Here's how the part is built. I have some questions about the finished solid (model axes, mm). A direction names the side the tool comes from. Coordinates: 2 decimals unless noted, no trailing zeros. Order: outer loops, then holes, each group sorted by start corner. A loop starts at its lowest first (then second) coordinate and runs counter-clockwise, first axis right, second up. Notation, with made-up numbers: (76.25, 47.25) - (106.25, 47.25) arc R20 ccw to (106.25, 83.25) - close; hole circle Ø8 at (-20, 68.5). An arc over 180 degrees is marked (long way). Answer in a Markdown table with one row per item. Add a question column.
Item 1: Will these pins go through, and if not, where does the flat tip stop? pin 1 Ø0.8 at (y, z) = (1, 32) entering from -X; pin 2 Ø1.5 at (x, z) = (-7.5, 0.5) entering from +Y; pin 3 Ø0.6 at (x, y) = (-6, -0.5) entering from +Z; pin 4 Ø1 at (y, z) = (-0.5, -5) entering from +X (3 decimals).
Item 2: I want a section at A-A (x = -10). Please give me the cut outline in (y, z), plus the area to 3 significant figures.
Item 3: On a 3-axis mill with a long thin cutter (end or side, diameter ignored), from which of +Z, -Z, +X, -X, +Y, -Y can I reach the whole of each face in a straight line? I mean faces 1 (the flat face through (-20, 1, 70.612)), 2 (the flat face through (-27.773, -0.626, 26.551)), 3 (the flat face through (-20, -1.27, 35)). Say none if no direction works.
Item 4: I want a section at D-D (y = -0.6). Count the separate pieces of the cut face and the enclosed holes in it, plus the area to 3 significant figures.
Item 5: If I drill on line 1 along X through (y, z) = (2.05, 52); line 2 along X through (y, z) = (-0.9, -7.62) (1 decimal); line 3 along Z through (x, y) = (-27.5, 0.55), over which ranges is the centre line in solid material (lowest first)? Write a range as from..to.
Item 6: Thinking about a two-plate mould opening in X: for faces 4 (the flat face through (-20, 1, -1.27)), 5 (the flat face through (-40.64, 1, 35)), 6 (the cylindrical face through (-20.03, -0.63, -6.07)), which applies, +X half, -X half, draft (parallel to the pull), parting line (faces both ways), or undercut?
Item 7: I want a section at B-B (z = 61). Please give me the cut outline in (x, y), plus the area to 3 significant figures.
Item 8: I want a section at C-C (x = -3.5). Please give me the cut outline in (y, z).
```python
from build123d import *

# Parameters (mm, degrees)
SKETCH1_W           = 41.91
SKETCH1_H           = 71.882
SKETCH1_W_2         = 39.37
SKETCH1_H_2         = 69.342
BOSS_EXTRUDE4_DEPTH = 2.54
SKETCH5_W           = 46.99
SKETCH5_H           = 76.962
BOSS_EXTRUDE5_DEPTH = 1.27
CHAMFER4_SIZE       = 2.54
CUT_EXTRUDE1_DEPTH  = 2.54
FILLET1_R           = 2.54
SKETCH7_R           = 1.5875
BOSS_EXTRUDE6_DEPTH = 1.27


with BuildPart() as part:
    # Sketch1 → Boss-Extrude4 (new body)
    with BuildSketch(Plane(origin=(0, 0, 0), x_dir=(1, 0, 0), z_dir=(0, 1, 0))):
        with Locations((-19.685, -34.671)):
            Rectangle(SKETCH1_W, SKETCH1_H)
        with Locations((-19.685, -34.671)):
            Rectangle(SKETCH1_W_2, SKETCH1_H_2, mode=Mode.SUBTRACT)
    extrude(amount=BOSS_EXTRUDE4_DEPTH)

    # Sketch5 → Boss-Extrude5 (add)
    with BuildSketch(Plane.XZ):
        with Locations((-19.685, 34.671)):
            Rectangle(SKETCH5_W, SKETCH5_H)
    extrude(amount=BOSS_EXTRUDE5_DEPTH)

    # Chamfer4
    chamfer4_edges = [part.edges().sort_by_distance(p)[0] for p in [
        (-43.18, -0.635, 73.152),
        (-43.18, -0.635, -3.81),
        (3.81, -0.635, -3.81),
        (3.81, -0.635, 73.152),
    ]]
    chamfer(chamfer4_edges, length=CHAMFER4_SIZE)

    # Sketch6 → Cut-Extrude1 (cut)
    with BuildSketch(Plane(origin=(0, 0, 0), x_dir=(1, 0, 0), z_dir=(0, 1, 0))):
        Polygon((-36.83, -2.54), (-2.54, -2.54), (-19.685, -29.888964801), align=None)
        Polygon((-36.83, -12.104070398), (-36.83, -57.237929602), (-22.68284632, -34.671), align=None)
        Polygon((-36.83, -66.802), (-2.54, -66.802), (-19.685, -39.453035199), align=None)
        Polygon((-2.54, -12.104070398), (-2.54, -57.237929602), (-16.68715368, -34.671), align=None)
    extrude(amount=-CUT_EXTRUDE1_DEPTH, mode=Mode.SUBTRACT)

    # Fillet1
    fillet1_edges = [part.edges().sort_by_distance(p)[0] for p in [
        (-2.54, -0.635, 2.54),
        (-19.685, -0.635, 29.888964801),
        (-36.83, -0.635, 2.54),
        (-36.83, -0.635, 66.802),
        (-19.685, -0.635, 39.453035199),
        (-2.54, -0.635, 66.802),
        (-22.68284632, -0.635, 34.671),
        (-36.83, -0.635, 57.237929602),
        (-36.83, -0.635, 12.104070398),
        (-16.68715368, -0.635, 34.671),
        (-2.54, -0.635, 12.104070398),
        (-2.54, -0.635, 57.237929602),
    ]]
    fillet(fillet1_edges, radius=FILLET1_R)

    # Sketch7 → Boss-Extrude6 (add)
    with BuildSketch(Plane(origin=(0, 0, 0), x_dir=(1, 0, 0), z_dir=(0, 1, 0))):
        with BuildLine():
            Line((-14.605, 7.62), (-14.605, 3.81))
            Line((-14.605, 3.81), (-24.765, 3.81))
            Line((-24.765, 3.81), (-24.765, 7.62))
            ThreePointArc((-24.765, 7.62), (-19.685, 12.7), (-14.605, 7.62))
        make_face()
        with Locations((-19.685, 7.62)):
            Circle(SKETCH7_R, mode=Mode.SUBTRACT)
        with BuildLine():
            Line((-24.765, -73.152), (-24.765, -76.962))
            ThreePointArc((-24.765, -76.962), (-19.685, -82.042), (-14.605, -76.962))
            Line((-14.605, -76.962), (-14.605, -73.152))
            Line((-14.605, -73.152), (-24.765, -73.152))
        make_face()
        with Locations((-19.685, -76.962)):
            Circle(SKETCH7_R, mode=Mode.SUBTRACT)
    extrude(amount=-BOSS_EXTRUDE6_DEPTH)


solid = part.part
```
Values follow:
| question | item | result |
|---|---|---|
| 1 | pin 1 | stops at x = -40.64 |
| 1 | pin 2 | stops at y = 2.54 |
| 1 | pin 3 | stops at z = 73.15 |
| 1 | pin 4 | stops at x = -14.605 |
| 2 | outline | (-1.27, -3.81) - (0, -3.81) - (0, -1.27) - (2.54, -1.27) - (2.54, 0) - (0, 0) - (0, 2.54) - (-1.27, 2.54) - close; (-1.27, 14.44) - (0, 14.44) - (0, 24) - (-1.27, 24) - close; (-1.27, 45.34) - (0, 45.34) - (0, 54.9) - (-1.27, 54.9) - close; (-1.27, 66.8) - (0, 66.8) - (0, 69.34) - (2.54, 69.34) - (2.54, 70.61) - (0, 70.61) - (0, 73.15) - (-1.27, 73.15) - close |
| 2 | area | 46.9 mm^2 |
| 3 | face 1 | +Z, +X, -X, +Y |
| 3 | face 2 | +Y, -Y |
| 3 | face 3 | +Z, -Z, +X, -X, -Y |
| 4 | separate pieces | 1 |
| 4 | enclosed holes | 6 |
| 4 | area | 2,250 mm^2 |
| 5 | line 1 | x = -40.64..-39.37, 0..1.27 |
| 5 | line 2 | x = -24.8..-21.3, -18.1..-14.6 |
| 5 | line 3 | z = -1.27..0, 69.34..70.61 |
| 6 | face 4 | draft |
| 6 | face 5 | -X half |
| 6 | face 6 | undercut |
| 7 | outline | (-43.18, -1.27) - (-33.19, -1.27) - (-33.19, 0) - (-39.37, 0) - (-39.37, 2.54) - (-40.64, 2.54) - (-40.64, 0) - (-43.18, 0) - close; (-6.18, -1.27) - (3.81, -1.27) - (3.81, 0) - (1.27, 0) - (1.27, 2.54) - (0, 2.54) - (0, 0) - (-6.18, 0) - close |
| 7 | area | 31.8 mm^2 |
| 8 | outline | (-1.27, -3.81) - (0, -3.81) - (0, -1.27) - (2.54, -1.27) - (2.54, 0) - (0, 0) - (0, 18.95) - (-1.27, 18.95) - close; (-1.27, 50.39) - (0, 50.39) - (0, 69.34) - (2.54, 69.34) - (2.54, 70.61) - (0, 70.61) - (0, 73.15) - (-1.27, 73.15) - close |
